```python
from build123d import *

# Parameters (mm, degrees)
EXTRUDE_1_DEPTH            = 5
SKETCH_16_W                = 130
SKETCH_16_H                = 20
CUT_EXTRUDE_16_DEPTH       = 10
CUT_EXTRUDE_START          = -6
SKETCH_9_R                 = 2.6
CUT_EXTRUDE_8_DEPTH        = 7
SKETCH_18_R                = 2.1
CUT_EXTRUDE_17_DEPTH       = 5
PATTERN_CIRCULAR_1_COUNT   = 3
CHAMFER_4_SIZE             = 5
SKETCH_5_R                 = 2.1
CUT_EXTRUDE_5_DEPTH        = 6
CUT_EXTRUDE_7_DEPTH        = 6
CHAMFER_2_SIZE             = 5
CHAMFER_2_OF_MIRROR_1_SIZE = 5
FILLET_2_R                 = 15
FILLET_3_R                 = 10


with BuildPart() as part:
    # 草圖1 → 填料-伸長1 (new body)
    with BuildSketch(Plane(origin=(0, 0, 0), x_dir=(1, 0, 0), z_dir=(0, 1, 0))):
        Polygon((85, 147.224318643), (-85, 147.224318643), (-170, 0), (-85, -147.224318643), (85, -147.224318643), (170, 0), align=None)
    extrude(amount=EXTRUDE_1_DEPTH)

    # 草圖16 → 除料-伸長16 (cut)
    with BuildSketch(Plane(origin=(0, 5, 0), x_dir=(1, 0, 0), z_dir=(0, 1, 0))):
        with Locations((0, -137.224318643)):
            Rectangle(SKETCH_16_W, SKETCH_16_H)
    cut_extrude_16 = extrude(amount=-CUT_EXTRUDE_16_DEPTH, mode=Mode.SUBTRACT)

    # 草圖9 → 除料-伸長8 (cut)
    with BuildSketch(Plane(origin=(0, 5, 0), x_dir=(1, 0, 0), z_dir=(0, 1, 0)).offset(CUT_EXTRUDE_START)):
        with Locations((-27.5, -119.224318643)):
            Circle(SKETCH_9_R)
        with Locations((-27.5, -107.224318643)):
            Circle(SKETCH_9_R)
        with Locations((27.5, -107.224318643)):
            Circle(SKETCH_9_R)
        with Locations((27.5, -119.224318643)):
            Circle(SKETCH_9_R)
    cut_extrude_8 = extrude(amount=CUT_EXTRUDE_8_DEPTH, mode=Mode.SUBTRACT)

    # 草圖18 → 除料-伸長17 (cut)
    with BuildSketch(Plane(origin=(0, 5, 0), x_dir=(1, 0, 0), z_dir=(0, 1, 0))):
        with Locations((-10, -69.224318643)):
            Circle(SKETCH_18_R)
        with Locations((10, -69.224318643)):
            Circle(SKETCH_18_R)
    cut_extrude_17 = extrude(amount=-CUT_EXTRUDE_17_DEPTH, mode=Mode.SUBTRACT)

    # 環狀複製排列1: 除料-伸長16, 除料-伸長8, 除料-伸長17 ×3 about axis
    pattern_circular_1_axis = Axis((0, 0, 0), (0, 1, 0))
    for i in range(1, PATTERN_CIRCULAR_1_COUNT):
        add(cut_extrude_16.rotate(pattern_circular_1_axis, i * 360 / PATTERN_CIRCULAR_1_COUNT), mode=Mode.SUBTRACT)
        add(cut_extrude_8.rotate(pattern_circular_1_axis, i * 360 / PATTERN_CIRCULAR_1_COUNT), mode=Mode.SUBTRACT)
        add(cut_extrude_17.rotate(pattern_circular_1_axis, i * 360 / PATTERN_CIRCULAR_1_COUNT), mode=Mode.SUBTRACT)

    # 導角4
    chamfer_4_edges = [part.edges().sort_by_distance(p)[0] for p in [
        (-65, 2.5, 147.224318643),
        (-65, 2.5, 127.224318643),
        (65, 2.5, 127.224318643),
        (65, 2.5, 147.224318643),
        (-95, 2.5, -129.903810568),
        (-77.679491924, 2.5, -119.903810568),
        (-142.679491924, 2.5, -7.320508076),
        (-160, 2.5, -17.320508076),
        (160, 2.5, -17.320508076),
        (142.679491924, 2.5, -7.320508076),
        (77.679491924, 2.5, -119.903810568),
        (95, 2.5, -129.903810568),
    ]]
    chamfer(chamfer_4_edges, length=CHAMFER_4_SIZE)

    # 草圖5 → 除料-伸長5 (cut, through all)
    with BuildSketch(Plane(origin=(0, 5, 0), x_dir=(1, 0, 0), z_dir=(0, 1, 0))):
        with Locations((-84.5, -112)):
            Circle(SKETCH_5_R)
        with Locations((-69.5, -112)):
            Circle(SKETCH_5_R)
        with Locations((84.5, -112)):
            Circle(SKETCH_5_R)
        with Locations((69.5, -112)):
            Circle(SKETCH_5_R)
    extrude(amount=-CUT_EXTRUDE_5_DEPTH, mode=Mode.SUBTRACT)

    # 草圖8 → 除料-伸長7 (cut, through all)
    with BuildSketch(Plane(origin=(0, 5, 0), x_dir=(1, 0, 0), z_dir=(0, 1, 0))):
        Polygon((-127.679491924, -33.301270189), (-97.679491924, -85.262794416), (-58.708348754, -62.762794416), (-88.708348754, -10.801270189), align=None)
    cut_extrude_7 = extrude(amount=-CUT_EXTRUDE_7_DEPTH, mode=Mode.SUBTRACT)

    # 導角2
    chamfer_2_edges = [part.edges().sort_by_distance(p)[0] for p in [
        (-127.679491924, 2.5, 33.301270189),
        (-88.708348754, 2.5, 10.801270189),
        (-58.708348754, 2.5, 62.762794416),
        (-97.679491924, 2.5, 85.262794416),
    ]]
    chamfer(chamfer_2_edges, length=CHAMFER_2_SIZE)

    # 鏡射1: 除料-伸長7 across plane
    add(cut_extrude_7.mirror(Plane(origin=(0, 0, 0), x_dir=(0, 0, 1), z_dir=(1, 0, 0))), mode=Mode.SUBTRACT)

    # 導角2 of 鏡射1
    chamfer_2_of_mirror_1_edges = [part.edges().sort_by_distance(p)[0] for p in [
        (127.679491924, 2.5, 33.301270189),
        (88.708348754, 2.5, 10.801270189),
        (58.708348754, 2.5, 62.762794416),
        (97.679491924, 2.5, 85.262794416),
    ]]
    chamfer(chamfer_2_of_mirror_1_edges, length=CHAMFER_2_OF_MIRROR_1_SIZE)

    # 圓角2
    fillet_2_edges = [part.edges().sort_by_distance(p)[0] for p in [
        (170, 2.5, 0),
        (85, 2.5, 147.224318643),
        (-85, 2.5, 147.224318643),
        (-170, 2.5, 0),
    ]]
    fillet(fillet_2_edges, radius=FILLET_2_R)

    # 圓角3
    fillet_3_edges = [part.edges().sort_by_distance(p)[0] for p in [
        (-85, 2.5, -147.224318643),
        (85, 2.5, -147.224318643),
    ]]
    fillet(fillet_3_edges, radius=FILLET_3_R)


solid = part.part
```
Could you check a few things on this model? Use its own coordinates, in mm. A direction names the side the tool comes from. Coordinates: 2 decimals unless noted, no trailing zeros. Write each loop counter-clockwise with the first axis right and the second up, starting at its lowest first coordinate (ties: lowest second). Pieces come first, ordered by that corner, then holes. Notation, with made-up numbers: (46, 89.25) -> (74, 89.25) arc R9 ccw to (74, 106.25) -> close; hole circle Ø8 at (71.5, 81.5). An arc over 180 degrees is marked (long way). One line per question, with ' | ' between items. Start each with the question number.
1. If we section it at B-B (x = -17): Please give me the cut outline in (y, z), and give its area (3 significant figures).
2. If we section it at C-C (y = 3.7): Count the separate pieces of the cut face and the enclosed holes in it, and give its area (3 significant figures).
3. Please list where these lines run through material, in increasing order: line 1 along X through (y, z) = (3.4, 37); line 2 along X through (y, z) = (3.55, 41); line 3 along Z through (x, y) = (-51, 1.85).
4. Thinking about a two-plate mould opening in Z: for faces 1 (the face through (83.74, 2.54, 145.27)), 2 (the face through (-2, 5, -2)), 3 (the face through (107.98, 2.54, 21.93)), which applies, pulls with the +Z half, pulls with the -Z half, needs draft (parallel to the pull), parting line crosses it, or undercut?
5. Will these pins go through, and if not, where does the flat tip stop? P1, Ø1.5, axis at y = 2.5, z = 139, coming from the -X side; P2, Ø2, axis at y = 0.5, z = 64, coming from the +X side; P3, Ø4, axis at x = 27.5, z = 107.22, coming from the +Y side; P4, Ø2.5, axis at y = 1.5, z = 136, coming from the +X side.
6. For faces 4 (the face through (-107.98, 2.54, 21.93)), 5 (the face through (-2, 0, -2)), which set-ups out of +Z, -Z, +X, -X, +Y, -Y let a thin tool reach every point of the face, with its end or its side?
7. If we section it at A-A (z = 77): Please give me the cut outline in (x, y).
8. If we section it at D-D (z = -65): Please give me the cut outline in (x, y), and give its area (3 significant figures).
Return value:
1) outline: (0, -147.22) -> (5, -147.22) -> (5, 127.22) -> (0, 127.22) -> close | area: 1,370 mm²
2) separate pieces: 1 | enclosed holes: 24 | area: 61,500 mm²
3) line 1: x = -148.64 to -125.01, -73.58 to 73.58, 125.01 to 148.64 | line 2: x = -146.33 to -123.23, -71.27 to 71.27, 123.23 to 146.33 | line 3: z = -147.22 to 127.22
4) face 1: pulls with the +Z half | face 2: needs draft | face 3: undercut
5) P1: stops at x = -90.18 | P2: stops at x = 133.63 | P3: passes through | P4: stops at x = 92.2
6) face 4: +Y, -Y | face 5: +Z, -Z, +X, -X, -Y
7) outline: (-125.54, 0) -> (-102.45, 0) -> (-102.45, 5) -> (-125.54, 5) -> close; (-83.37, 0) -> (83.37, 0) -> (83.37, 5) -> (-83.37, 5) -> close; (102.45, 0) -> (125.54, 0) -> (125.54, 5) -> (102.45, 5) -> close
8) outline: (-109.38, 0) -> (109.38, 0) -> (109.38, 5) -> (-109.38, 5) -> close | area: 1,090 mm²
